Verification items for the finished model (mm, model axes). A direction names the side the tool comes from. Round coordinates to 2 decimals unless told otherwise and drop trailing zeros. Loops run counter-clockwise (first coordinate to the right, second up) from the corner with the lowest first, then second, coordinate; pieces in that order, holes last. Notation, with made-up numbers: (21, 14) -> (32, 14) arc R28 ccw to (32, 32) -> close; hole circle Ø6 at (80, 62.25). An arc over 180 degrees is marked (long way). Write item = value, one per line. Start each with the question number.
```python
from build123d import *

# Parameters (mm, degrees)
SKETCH1_R               = 2
BOSS_EXTRUDE1_DEPTH     = 16
CHAMFER1_SIZE           = 0.5
SKETCH7_R               = 1
CUT_EXTRUDE1_DEPTH      = 4.305898307
CUT_EXTRUDE1_DEPTH_BACK = 4.305898307


with BuildPart() as part:
    # Sketch1 → Boss-Extrude1 (new body)
    with BuildSketch(Plane.XY):
        Circle(SKETCH1_R)
    extrude(amount=-BOSS_EXTRUDE1_DEPTH)

    # Chamfer1
    chamfer1_edges = [part.edges().sort_by_distance(p)[0] for p in [
        (-2, 0, 0),
    ]]
    chamfer(chamfer1_edges, length=CHAMFER1_SIZE)

    # Sketch4 → Revolve1 (revolve)
    with BuildSketch(Plane(origin=(0, 0, 0), x_dir=(0, 0, -1), z_dir=(1, 0, 0))):
        with BuildLine():
            Line((16, 0), (16, 3.305898307))
            ThreePointArc((16, 3.305898307), (17.582389504, 1.978570239), (18.174855662, 0))
            Line((18.174855662, 0), (16, 0))
        make_face()
    revolve(axis=Axis((0, 0, -13.297823311), (0, 0, -1)))

    # Sketch7 → Cut-Extrude1 (cut, two sides)
    with BuildSketch(Plane(origin=(0, 0, 0), x_dir=(0, 0, -1), z_dir=(1, 0, 0))) as cut_extrude1_sk:
        with Locations((2.5, 0)):
            Circle(SKETCH7_R)
    extrude(amount=CUT_EXTRUDE1_DEPTH, mode=Mode.SUBTRACT)
    extrude(cut_extrude1_sk.sketch, amount=-CUT_EXTRUDE1_DEPTH_BACK, mode=Mode.SUBTRACT)


solid = part.part
```
(1) Section check C-C on z = -8.5. Enter the section's corners in (x, y), then the cut area to 3 significant figures.
(2) Access from +Z, -Z, +X, -X, +Y, -Y to the whole of each face (thin tool, end or side, straight path). Record for faces 1 (the flat face through (0, 0, 0)), 2 (the cylindrical face through (-2, 0, -8)).
(3) Section check A-A on y = 0. Enter the section's corners in (x, z), then the cut area to 3 significant figures.
(4) Scan lines: line 1 (Z direction, x = -1, y = 0.75); line 2 (Z direction, x = 0.8, y = 0); line 3 (X direction, y = 0, z = -12). Record each from-to range of solid material in increasing order. Write a range as [from, to].
(5) Depth check by flat-ended pin: pin 1 Ø1.5 at (x, z) = (1.5, -5) entering from -Y; pin 2 Ø2 at (y, z) = (2.5, -10) entering from -X; pin 3 Ø1.6 at (y, z) = (0, -2.5) entering from -X; pin 4 Ø2 at (y, z) = (-1.5, -10.5) entering from -X. Enter the tip coordinate at first touch or a pass-through.
(6) Section check B-B on z = -2.5. Enter the section's corners in (x, y).
(7) Section check D-D on x = 2.25. Enter the section's corners in (y, z), then the cut area to 3 significant figures.
Computed values:
q1.outline = circle Ø4 at (0, 0)
q1.area = 12.6 mm²
q2.face_1 = +Z, +X, -X, +Y, -Y
q2.face_2 = +Z
q3.outline = (-3.31, -16) arc R3.6 ccw to (3.31, -16) -> (2, -16) -> (2, -3.5) -> (-2, -3.5) -> (-2, -16) -> close; (-2, -1.5) -> (2, -1.5) -> (2, -0.5) -> (1.5, 0) -> (-1.5, 0) -> (-2, -0.5) -> close
q3.area = 66.1 mm²
q4.line_1 = [-17.95, -3.16], [-1.84, 0]
q4.line_2 = [-18.08, -3.5], [-1.5, 0]
q4.line_3 = [-2, 2]
q5.pin_1 = -1.85
q5.pin_2 = -1.32
q5.pin_3 = through
q5.pin_4 = -1.94
q6.outline = (-1.73, -1) arc R2 ccw to (1.73, -1) -> close; (-1.73, 1) -> (1.73, 1) arc R2 ccw to start
q7.outline = (-2.42, -16) arc R2.81 ccw to (2.42, -16) -> close
q7.area = 4.75 mm²
